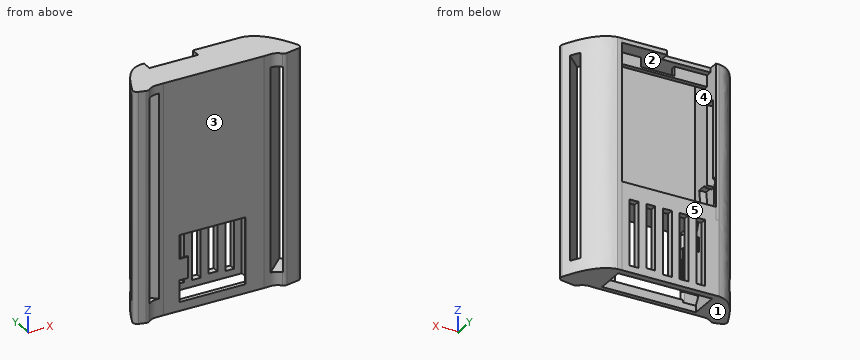
```python
from build123d import *

# Parameters (mm, degrees)
BOSS_EXTRUDE2_DEPTH      = 52
FILLET2_R                = 1
CUT_EXTRUDE2_DEPTH       = 3
CUT_EXTRUDE2_DEPTH_BACK  = 6
SKETCH10_W               = 2.350757351
SKETCH10_H               = 46
SKETCH11_W               = 17
SKETCH11_H               = 15
PELTIER_DEPTH            = 10
SKETCH12_W               = 21
SKETCH12_H               = 29
BATTERY_DEPTH            = 0.4
SKETCH14_W               = 21.3
SKETCH14_H               = 1
BOSS_EXTRUDE4_DEPTH      = 7.999920354
SKETCH15_W               = 3.297714658
SKETCH15_H               = 0.629450307
CUT_EXTRUDE5_DEPTH       = 3.6
SKETCH16_W               = 2.795507754
SKETCH16_H               = 0.669410668
CUT_EXTRUDE6_DEPTH       = 4.337027413
FILLET3_R                = 1
CUT_EXTRUDE7_DEPTH       = 1.6
CUT_EXTRUDE8_DEPTH       = 1.6
FILLET4_R                = 1
FILLET5_R                = 1
SKETCH19_W               = 21.3
SKETCH19_H               = 1
BOSS_EXTRUDE5_DEPTH      = 2.6
SKETCH20_W               = 7.625924169
SKETCH20_H               = 2.120993271
CUT_EXTRUDE9_DEPTH       = 2.6
SKETCH21_W               = 21.3
SKETCH21_H               = 2.886084762
BOSS_EXTRUDE6_DEPTH      = 8
SKETCH22_W               = 17
SKETCH22_H               = 1.5
BOSS_EXTRUDE7_DEPTH      = 22
SKETCH23_W               = 24.481547991
SKETCH23_H               = 2.403526745
CUT_EXTRUDE10_DEPTH      = 2
SKETCH24_W               = 15
SKETCH24_H               = 0.211445756
BOSS_EXTRUDE8_DEPTH      = 2
SKETCH25_W               = 4.787241237
SKETCH25_H               = 0.237383131
BOSS_EXTRUDE9_DEPTH      = 2
SKETCH26_W               = 11.036128308
SKETCH26_H               = 2.126226966
CUT_EXTRUDE11_DEPTH      = 2
CUT_EXTRUDE12_DEPTH      = 2
CUT_EXTRUDE12_DEPTH_BACK = 11
SKETCH27_W               = 46
SKETCH27_H               = 2.33
SKETCH28_W               = 1.978966
SKETCH28_H               = 14.822133623
SKETCH28_H_2             = 14.389327905
SKETCH28_W_2             = 1.978965999
CUT_EXTRUDE13_DEPTH      = 3
SKETCH29_W               = 3.210088646
SKETCH29_H               = 7.129450307
CUT_EXTRUDE14_DEPTH      = 7


with BuildPart() as part:
    # Sketch1 → Boss-Extrude2 (new body)
    with BuildSketch(Plane.XY):
        with BuildLine():
            Line((-4.066957942, -1.190846618), (-7.240355005, -0.354620493))
            add(Edge.make_bspline(
                [(0.042333709, 8.998333002), (-4.213116867, 8.648828695), (-5.962383558, 1.81462105), (-7.240355005, -0.354620493)],
                knots=[0, 0, 0, 0, 1, 1, 1, 1], degree=3))
            Line((0.042333709, 8.998333002), (0.742333709, 8.998333002))
            Line((0.742333709, 8.998333002), (0.742333709, 1))
            Line((0.742333709, 1), (22.042333709, 1))
            Line((22.042333709, 1), (22.042333709, 8.998333002))
            Line((22.042333709, 8.998333002), (23.042333709, 8.998333002))
            add(Edge.make_bspline(
                [(23.042333709, 8.998333002), (27.852391375, 8.27132168), (31.467788923, -0.354620493)],
                knots=[0, 0, 0, 1, 1, 1], degree=2))
            Line((31.467788923, -0.354620493), (26.875523276, -1.190846618))
            add(Edge.make_bspline(
                [(22.86911945, 0), (24.564241842, 0.074416087), (25.297281614, 0.429058332), (26.875523276, -1.190846618)],
                knots=[0, 0, 0, 0, 1, 1, 1, 1], degree=3))
            Line((22.86911945, 0), (0, 0))
            add(Edge.make_bspline(
                [(0, 0), (-1.870814346, -0.163675047), (-2.239916233, 0.430706612), (-4.066957942, -1.190846618)],
                knots=[0, 0, 0, 0, 1, 1, 1, 1], degree=3))
        make_face()
    extrude(amount=BOSS_EXTRUDE2_DEPTH)

    # Fillet2
    fillet2_edges = [part.edges().sort_by_distance(p)[0] for p in [
        (-4.066957942, -1.190846618, 26),
        (-7.240355005, -0.354620493, 26),
    ]]
    fillet(fillet2_edges, radius=FILLET2_R)

    # Sketch10 → Cut-Extrude2 (cut, two sides: drawn at the far end of the back side and taken through both)
    with BuildSketch(Plane(origin=(-4.380890916, 3.569201652, 0), x_dir=(0.631629007569502, 0.7752707893354205, 0), z_dir=(-0.7752707893354205, 0.631629007569502, 0)).offset(-CUT_EXTRUDE2_DEPTH_BACK)):
        with Locations((-1.831509184, -27)):
            Rectangle(SKETCH10_W, SKETCH10_H)
    extrude(amount=CUT_EXTRUDE2_DEPTH + CUT_EXTRUDE2_DEPTH_BACK, mode=Mode.SUBTRACT)

    # Sketch11 → Peltier (cut)
    with BuildSketch(Plane(origin=(0, 1, 0), x_dir=(1, 0, 0), z_dir=(0, 1, 0))):
        with Locations((12.114692368, -9.5)):
            Rectangle(SKETCH11_W, SKETCH11_H)
    extrude(amount=-PELTIER_DEPTH, mode=Mode.SUBTRACT)

    # Sketch12 → Battery (cut)
    with BuildSketch(Plane(origin=(0, 1, 0), x_dir=(1, 0, 0), z_dir=(0, 1, 0))):
        with Locations((11.242333709, -36.5)):
            Rectangle(SKETCH12_W, SKETCH12_H)
    extrude(amount=-BATTERY_DEPTH, mode=Mode.SUBTRACT)

    # Sketch14 → Boss-Extrude4 (add)
    with BuildSketch(Plane(origin=(0, 1, 0), x_dir=(1, 0, 0), z_dir=(0, 1, 0))):
        with Locations((11.392333709, -51.5)):
            Rectangle(SKETCH14_W, SKETCH14_H)
    extrude(amount=BOSS_EXTRUDE4_DEPTH)

    # Sketch15 → Cut-Extrude5 (cut)
    with BuildSketch(Plane(origin=(3.614692368, 0, 0), x_dir=(0, 0, -1), z_dir=(1, 0, 0))):
        with Locations((-15.351142671, 0.685274847)):
            Rectangle(SKETCH15_W, SKETCH15_H)
    extrude(amount=-CUT_EXTRUDE5_DEPTH, mode=Mode.SUBTRACT)

    # Sketch16 → Cut-Extrude6 (cut)
    with BuildSketch(Plane(origin=(3.614692368, 0, 0), x_dir=(0, 0, -1), z_dir=(1, 0, 0))):
        with Locations((-2.862635658, 0.665294666)):
            Rectangle(SKETCH16_W, SKETCH16_H)
    extrude(amount=-CUT_EXTRUDE6_DEPTH, mode=Mode.SUBTRACT)

    # Fillet3
    # the kernel refuses this fillet: 1 mm, written as the material it takes off along each edge
    with BuildSketch(Plane(origin=(3.614692368, 0.330589332, 2), x_dir=(0, -1, 0), z_dir=(0, 0, 1))) as fillet3_piece_1:
        with BuildLine():
            CenterArc((1, -0.742892561), FILLET3_R, 132.021596152, 47.978403848)
            Line((0, -0.742892561), (0, 0))
            Line((0, 0), (0.330589332, 0))
        make_face()
    extrude(amount=2.260389535, mode=Mode.SUBTRACT)
    with BuildSketch(Plane(origin=(3.614692368, 0.370549693, 17), x_dir=(0, -1, 0), z_dir=(0, 0, -1))) as fillet3_piece_2:
        with BuildLine():
            CenterArc((1, 0.77704074), FILLET3_R, 180, 50.990421184)
            Line((0, 0.77704074), (0, 0))
            Line((0, 0), (0.370549693, 0))
        make_face()
    extrude(amount=3.297714658, mode=Mode.SUBTRACT)

    # Sketch17 → Cut-Extrude7 (cut)
    with BuildSketch(Plane(origin=(0.742333709, 0, 0), x_dir=(0, 0, -1), z_dir=(1, 0, 0))):
        with BuildLine():
            Line((-26.679947222, 8.607264172), (-26.2562675, 4.600305927))
            add(Edge.make_bspline(
                [(-11.956359989, 1), (-18.174048642, 5.645894808), (-26.2562675, 4.600305927)],
                knots=[0, 0, 0, 1, 1, 1], degree=2))
            Line((-11.956359989, 1), (-1.464881781, 1))
            add(Edge.make_bspline(
                [(-1.464881781, 1), (-12.835212302, 8.374655541), (-26.679947222, 8.607264172)],
                knots=[0, 0, 0, 1, 1, 1], degree=2))
        make_face()
    extrude(amount=-CUT_EXTRUDE7_DEPTH, mode=Mode.SUBTRACT)

    # Sketch18 → Cut-Extrude8 (cut)
    with BuildSketch(Plane(origin=(0.742333709, 0, 0), x_dir=(0, 0, -1), z_dir=(1, 0, 0))):
        with BuildLine():
            Line((-26.709406335, 2.333242891), (-26.709406335, 4.472060633))
            add(Edge.make_bspline(
                [(-10.082290903, 1), (-18.147687182, 7.131693783), (-26.709406335, 4.472060633)],
                knots=[0, 0, 0, 1, 1, 1], degree=2))
            Line((-10.082290903, 1), (-17, 1))
            add(Edge.make_bspline(
                [(-17, 1), (-21.703390607, 3.354733642), (-26.709406335, 2.333242891)],
                knots=[0, 0, 0, 1, 1, 1], degree=2))
        make_face()
    extrude(amount=-CUT_EXTRUDE8_DEPTH, mode=Mode.SUBTRACT)

    # Fillet4
    fillet4_edges = [part.edges().sort_by_distance(p)[0] for p in [
        (26.875523276, -1.190846618, 26),
    ]]
    fillet(fillet4_edges, radius=FILLET4_R)

    # Fillet5
    fillet5_edges = [part.edges().sort_by_distance(p)[0] for p in [
        (31.467788923, -0.354620493, 26),
    ]]
    fillet(fillet5_edges, radius=FILLET5_R)

    # Sketch19 → Boss-Extrude5 (add)
    with BuildSketch(Plane(origin=(0, 0, 51), x_dir=(-1, 0, 0), z_dir=(0, 0, -1))):
        with Locations((-11.392333709, 5)):
            Rectangle(SKETCH19_W, SKETCH19_H)
    extrude(amount=BOSS_EXTRUDE5_DEPTH)

    # Sketch20 → Cut-Extrude9 (cut)
    with BuildSketch(Plane(origin=(0, 5.5, 0), x_dir=(1, 0, 0), z_dir=(0, 1, 0))):
        with Locations((11.936871332, -49.939503364)):
            Rectangle(SKETCH20_W, SKETCH20_H)
    extrude(amount=-CUT_EXTRUDE9_DEPTH, mode=Mode.SUBTRACT)

    # Sketch21 → Boss-Extrude6 (add)
    with BuildSketch(Plane(origin=(0, 1, 0), x_dir=(1, 0, 0), z_dir=(0, 1, 0))):
        with Locations((11.392333709, -18.443042381)):
            Rectangle(SKETCH21_W, SKETCH21_H)
    extrude(amount=BOSS_EXTRUDE6_DEPTH)

    # Sketch22 → Boss-Extrude7 (add)
    with BuildSketch(Plane.ZY.offset(-22.042333709)):
        with Locations((8.5, 8.25)):
            Rectangle(SKETCH22_W, SKETCH22_H)
    extrude(amount=BOSS_EXTRUDE7_DEPTH)

    # Sketch23 → Cut-Extrude10 (cut)
    with BuildSketch(Plane(origin=(0.742333709, 0, 0), x_dir=(0, 0, -1), z_dir=(1, 0, 0))):
        with Locations((-32.126858758, 6.701763373)):
            Rectangle(SKETCH23_W, SKETCH23_H)
    extrude(amount=-CUT_EXTRUDE10_DEPTH, mode=Mode.SUBTRACT)

    # Sketch24 → Boss-Extrude8 (add)
    with BuildSketch(Plane.ZY.offset(-20.614692368)):
        with Locations((9.5, 0.105722878)):
            Rectangle(SKETCH24_W, SKETCH24_H)
    extrude(amount=BOSS_EXTRUDE8_DEPTH)

    # Sketch25 → Boss-Extrude9 (add)
    with BuildSketch(Plane(origin=(3.614692368, 0, 0), x_dir=(0, 0, -1), z_dir=(1, 0, 0))):
        with Locations((-9.281203123, 0.118691566)):
            Rectangle(SKETCH25_W, SKETCH25_H)
    extrude(amount=BOSS_EXTRUDE9_DEPTH)

    # Sketch26 → Cut-Extrude11 (cut)
    with BuildSketch(Plane(origin=(0, 0, 51), x_dir=(-1, 0, 0), z_dir=(0, 0, -1))):
        with Locations((-6.260397863, 7.936806871)):
            Rectangle(SKETCH26_W, SKETCH26_H)
    extrude(amount=-CUT_EXTRUDE11_DEPTH, mode=Mode.SUBTRACT)

    # Sketch27 → Cut-Extrude12 (cut, two sides: drawn at the far end of the back side and taken through both)
    with BuildSketch(Plane(origin=(16.401330443, 15.864191281, 0), x_dir=(0, 0, -1), z_dir=(0.7187787233935905, 0.6952389134654938, 0)).offset(-CUT_EXTRUDE12_DEPTH_BACK)):
        with Locations((-26, -18.013212029)):
            Rectangle(SKETCH27_W, SKETCH27_H)
    extrude(amount=CUT_EXTRUDE12_DEPTH + CUT_EXTRUDE12_DEPTH_BACK, mode=Mode.SUBTRACT)

    # Sketch28 → Cut-Extrude13 (cut)
    with BuildSketch(Plane(origin=(0, 9, 0), x_dir=(1, 0, 0), z_dir=(0, 1, 0))):
        with Locations((19.299375066, -8.918059871)):
            Rectangle(SKETCH28_W, SKETCH28_H)
        with Locations((15.520409066, -9.13446273)):
            Rectangle(SKETCH28_W, SKETCH28_H_2)
        with Locations((11.741443067, -8.918059871)):
            Rectangle(SKETCH28_W_2, SKETCH28_H)
        with Locations((7.962477067, -8.918059871)):
            Rectangle(SKETCH28_W, SKETCH28_H)
        with Locations((4.183511067, -8.918059871)):
            Rectangle(SKETCH28_W, SKETCH28_H)
    extrude(amount=-CUT_EXTRUDE13_DEPTH, mode=Mode.SUBTRACT)

    # Sketch29 → Cut-Extrude14 (cut)
    with BuildSketch(Plane(origin=(0, 0, 17), x_dir=(-1, 0, 0), z_dir=(0, 0, -1))):
        with Locations((-2.347378032, 3.935274847)):
            Rectangle(SKETCH29_W, SKETCH29_H)
    extrude(amount=-CUT_EXTRUDE14_DEPTH, mode=Mode.SUBTRACT)


solid = part.part
```
Geometry: final body of the model. Coordinates: model frame, mm. Face numbers are marked on the shaded views. A direction names the side the tool comes from. Give positions to 0.01 mm unless a question says otherwise; leave off trailing zeros. Loops run counter-clockwise (first coordinate to the right, second up) from the corner with the lowest first, then second, coordinate; pieces in that order, holes last. Notation, with made-up numbers: (46, 23) - (85, 23) arc R15 ccw to (85, 47) - close; hole circle Ø5 at (5.25, 57.25). An arc over 180 degrees is marked (long way). Answer as CSV lines item,"result". Start each with the question number.
(1) Ray query, line 1 along Z through (x, y) = (13.5, 5.25); line 2 along Z through (x, y) = (-4, 0); line 3 along Y through (x, z) = (2.5, 7.5). Return the intervals inside material, ascending. Write a range as [from, to].
(2) Pin query (flat end, axial travel): P1, Ø0.5, axis at y = 5, z = 50.5, coming from the +X side; P2, Ø1.1, axis at x = 16.5, y = 5, coming from the -Z side; P3, Ø1.2, axis at x = 4.5, y = 8.5, coming from the +Z side. Return the tip coordinate at first contact, or that it passes through.
(3) Reachability of the marked faces 1, 2 and 3 from +Z, -Z, +X, -X, +Y, -Y: full face, straight path, thin tool, end or side. Return the list, or none.
(4) Section query B-B (z = 38.5). Give the number of separate pieces and of enclosed holes in the cut face, and give its area (3 significant figures).
(5) Section query A-A (x = 17.5). Output: boundary loops of the cut face in (y, z), and give its area (3 significant figures).
(6) Mould query, pull axis X, two halves, no side actions, for the marked faces 4 and 5. Classes: +X half, -X half, draft (parallel to the pull), parting line (faces both ways), or undercut.
Worked answers:
1,line 1,"z = [17, 19.89], [48.4, 48.88], [51, 52]"
1,line 2,"z = [0, 4], [50, 52]"
1,line 3,"y = [0, 1], [7.5, 9]"
2,P1,"stops at x = 28.77"
2,P2,"stops at z = 17"
2,P3,"stops at z = 19.89"
3,face 1,"-Z, +X, -X, +Y, -Y"
3,face 2,"none"
3,face 3,"+Z, -Z, -Y"
4,separate pieces,"3"
4,enclosed holes,"0"
4,area,"99.2 mm^2"
5,outline,"(0, 0) - (1, 0) - (1, 2) - (0, 2) - close; (0, 17) - (7.5, 17) - (7.5, 0) - (9, 0) - (9, 19.89) - (1, 19.89) - (1, 22) - (0.6, 22) - (0.6, 51) - (4.5, 51) - (4.5, 48.4) - (5.5, 48.4) - (5.5, 51) - (9, 51) - (9, 52) - (0, 52) - close"
5,area,"84.6 mm^2"
6,face 4,"undercut"
6,face 5,"draft"
